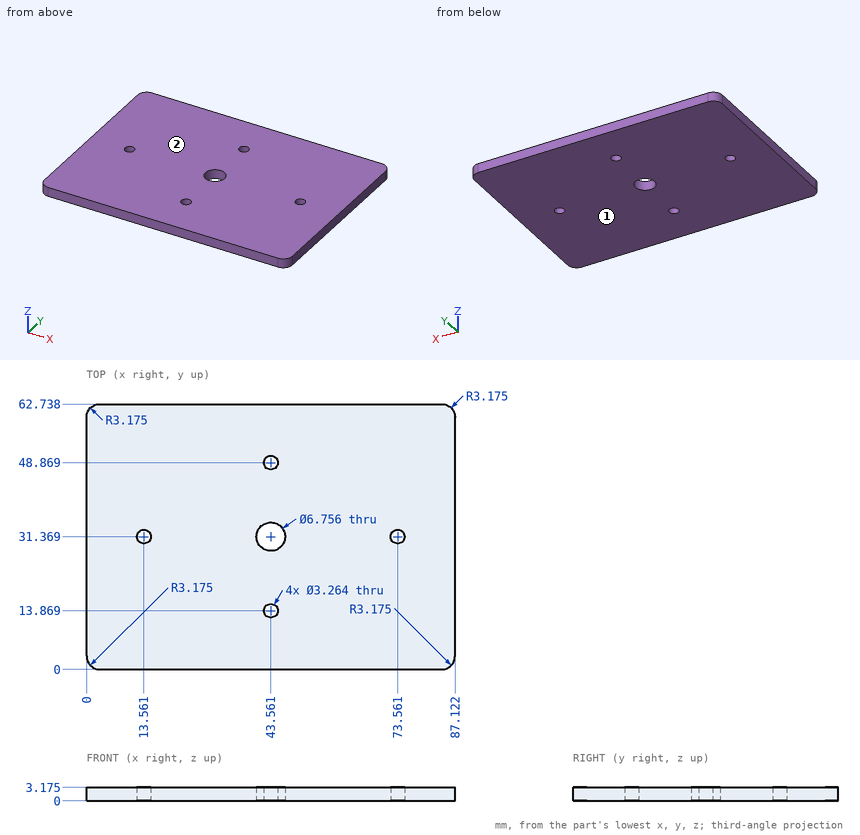
Job drawing, mm, ordinate dimensions from the low corner. One solid piece. Coordinates: 2 decimals unless noted, no trailing zeros. Answer in a Markdown table with one row per item. Add a question column.
Q1. Drop a flat-ended pin along its axis: pin 1 (3 mm diameter, centred on x = 73.561, y = 31.369, fed in from -Z). Give the stop position or say it passes through.
Q2. Mould opens along Z. For the marked faces 1 and 2 say: +Z half, -Z half, draft (parallel to the pull), parting line (faces both ways), or undercut.
Q3. Wall check: line 1 along Y through (x, z) = (12.5, 3.05); line 2 along Y through (x, z) = (14.5, 1.15) (1 decimal); line 3 along X through (y, z) = (48, 0.8). Give the ranges that are in metal, low to high. Write a range as [from, to].
Answers follow:
| question | item | result |
|---|---|---|
| 1 | pin 1 | through |
| 2 | face 1 | -Z half |
| 2 | face 2 | +Z half |
| 3 | line 1 | [0, 30.13], [32.61, 62.74] |
| 3 | line 2 | [0, 30], [32.7, 62.7] |
| 3 | line 3 | [0, 42.18], [44.94, 87.12] |
